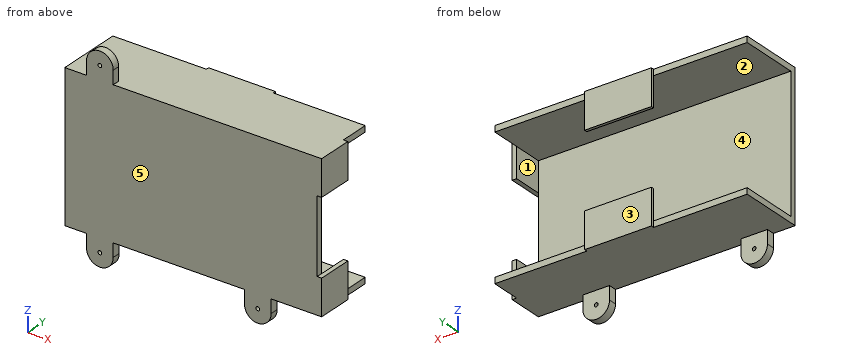
from build123d import *

# Parameters (mm, degrees)
SKETCH1_W           = 215.9
SKETCH1_H           = 114.3
BOSS_EXTRUDE1_DEPTH = 5.08
SKETCH2_W           = 215.9
SKETCH2_H           = 55.88
BOSS_EXTRUDE2_DEPTH = 5.08
SKETCH4_W           = 30.48
SKETCH4_H           = 30.48
BOSS_EXTRUDE3_DEPTH = 3.81
SKETCH5_W           = 57.15
SKETCH5_H           = 30.48
SKETCH5_W_2         = 57.169606557
BOSS_EXTRUDE4_DEPTH = 2.54
BOSS_EXTRUDE6_DEPTH = 15.875
SKETCH14_R          = 1.5875
CUT_EXTRUDE1_DEPTH  = 236.930487909
BOSS_EXTRUDE7_DEPTH = 15.875
SKETCH21_R          = 1.5875
CUT_EXTRUDE6_DEPTH  = 236.930487909
CUT_EXTRUDE10_START = -9.525
CUT_EXTRUDE10_DEPTH = 9.525
CUT_EXTRUDE11_START = -8.89
CUT_EXTRUDE11_DEPTH = 8.89
CUT_EXTRUDE12_START = -8.89
CUT_EXTRUDE12_DEPTH = 8.89


with BuildPart() as part:
    # Sketch1 → Boss-Extrude1 (new body)
    with BuildSketch(Plane(origin=(0, 0, 0), x_dir=(1, 0, 0), z_dir=(0, 1, 0))):
        with Locations((-107.95, 0)):
            Rectangle(SKETCH1_W, SKETCH1_H)
    extrude(amount=BOSS_EXTRUDE1_DEPTH)

    # Sketch2 → Boss-Extrude2 (add)
    with BuildSketch(Plane.XY.offset(57.15)):
        with Locations((-107.95, 27.94)):
            Rectangle(SKETCH2_W, SKETCH2_H)
    boss_extrude2 = extrude(amount=BOSS_EXTRUDE2_DEPTH)

    # Mirror1: Boss-Extrude2 across plane
    add(boss_extrude2.mirror(Plane.XY))

    # Sketch4 → Boss-Extrude3 (add)
    with BuildSketch(Plane(origin=(0, 0, 0), x_dir=(0, 0, -1), z_dir=(1, 0, 0))):
        with Locations((-46.99, 15.24)):
            Rectangle(SKETCH4_W, SKETCH4_H)
        with Locations((46.99, 15.24)):
            Rectangle(SKETCH4_W, SKETCH4_H)
    extrude(amount=BOSS_EXTRUDE3_DEPTH)

    # Sketch5 → Boss-Extrude4 (add)
    with BuildSketch(Plane(origin=(0, 55.88, 0), x_dir=(1, 0, 0), z_dir=(0, 1, 0))):
        with Locations((-107.309206557, 46.99)):
            Rectangle(SKETCH5_W, SKETCH5_H)
        with Locations((-107.299403278, -46.99)):
            Rectangle(SKETCH5_W_2, SKETCH5_H)
    extrude(amount=BOSS_EXTRUDE4_DEPTH)

    # Sketch12 → Boss-Extrude6 (add)
    with BuildSketch(Plane(origin=(0, 0, 0), x_dir=(1, 0, 0), z_dir=(0, 1, 0))):
        with BuildLine():
            Line((-62.23, 62.23), (-62.23, 73.66))
            ThreePointArc((-62.23, 73.66), (-50.8, 85.09), (-39.37, 73.66))
            Line((-39.37, 73.66), (-39.37, 62.23))
            Line((-39.37, 62.23), (-62.23, 62.23))
        make_face()
    extrude(amount=BOSS_EXTRUDE6_DEPTH)

    # Sketch14 → Cut-Extrude1 (cut, through all)
    with BuildSketch(Plane(origin=(0, 15.875, 0), x_dir=(1, 0, 0), z_dir=(0, 1, 0))):
        with Locations(Location((-50.8, 73.66, 0), (0, 0, 270))):
            Circle(SKETCH14_R)
    extrude(amount=-CUT_EXTRUDE1_DEPTH, mode=Mode.SUBTRACT)

    # Sketch20 → Boss-Extrude7 (add)
    with BuildSketch(Plane(origin=(0, 0, 0), x_dir=(1, 0, 0), z_dir=(0, 1, 0))):
        with BuildLine():
            Line((-197.317867116, 62.23), (-197.317867116, 73.66))
            ThreePointArc((-197.317867116, 73.66), (-185.887867116, 85.09), (-174.457867116, 73.66))
            Line((-174.457867116, 73.66), (-174.457867116, 62.23))
            Line((-174.457867116, 62.23), (-197.317867116, 62.23))
        make_face()
    boss_extrude7 = extrude(amount=BOSS_EXTRUDE7_DEPTH)

    # Sketch21 → Cut-Extrude6 (cut, through all)
    with BuildSketch(Plane(origin=(0, 15.875, 0), x_dir=(1, 0, 0), z_dir=(0, 1, 0))):
        with Locations(Location((-185.887867116, 73.66, 0), (0, 0, 270))):
            Circle(SKETCH21_R)
    cut_extrude6 = extrude(amount=-CUT_EXTRUDE6_DEPTH, mode=Mode.SUBTRACT)

    # Mirror4: Boss-Extrude7 across plane
    add(boss_extrude7.mirror(Plane.XY))

    # Mirror5: Cut-Extrude6 across plane
    add(cut_extrude6.mirror(Plane.XY), mode=Mode.SUBTRACT)

    # Sketch25 → Cut-Extrude10 (cut)
    with BuildSketch(Plane(origin=(0, 15.875, 0), x_dir=(1, 0, 0), z_dir=(0, 1, 0)).offset(CUT_EXTRUDE10_START)):
        with BuildLine():
            Line((-197.317867116, -62.23), (-197.317867116, -73.66))
            ThreePointArc((-197.317867116, -73.66), (-185.887867116, -85.09), (-174.457867116, -73.66))
            Line((-174.457867116, -73.66), (-174.457867116, -62.23))
            Line((-174.457867116, -62.23), (-197.317867116, -62.23))
        make_face()
    extrude(amount=CUT_EXTRUDE10_DEPTH, mode=Mode.SUBTRACT)

    # Sketch26 → Cut-Extrude11 (cut)
    with BuildSketch(Plane(origin=(0, 15.875, 0), x_dir=(1, 0, 0), z_dir=(0, 1, 0)).offset(CUT_EXTRUDE11_START)):
        with BuildLine():
            Line((-62.23, 62.23), (-39.37, 62.23))
            Line((-39.37, 62.23), (-39.37, 73.66))
            ThreePointArc((-39.37, 73.66), (-50.8, 85.09), (-62.23, 73.66))
            Line((-62.23, 73.66), (-62.23, 62.23))
        make_face()
    extrude(amount=CUT_EXTRUDE11_DEPTH, mode=Mode.SUBTRACT)

    # Sketch27 → Cut-Extrude12 (cut)
    with BuildSketch(Plane(origin=(0, 15.875, 0), x_dir=(1, 0, 0), z_dir=(0, 1, 0)).offset(CUT_EXTRUDE12_START)):
        with BuildLine():
            Line((-197.317867116, 62.23), (-174.457867116, 62.23))
            Line((-174.457867116, 62.23), (-174.457867116, 73.66))
            ThreePointArc((-174.457867116, 73.66), (-185.887867116, 85.09), (-197.317867116, 73.66))
            Line((-197.317867116, 73.66), (-197.317867116, 62.23))
        make_face()
    extrude(amount=CUT_EXTRUDE12_DEPTH, mode=Mode.SUBTRACT)


solid = part.part
Could you check a few things on this model? Use its own coordinates, in mm. Face numbers are marked on the shaded views. A direction names the side the tool comes from. Coordinates: 2 decimals unless noted, no trailing zeros. Order: outer loops, then holes, each group sorted by start corner. A loop starts at its lowest first (then second) coordinate and runs counter-clockwise, first axis right, second up. Notation, with made-up numbers: (-27, 74) -> (18, 74) arc R34 cw to (18, 108) -> close; hole circle Ø1 at (-18.5, -38.75). An arc over 180 degrees is marked (long way). One line per item, written item: value. Start each with the question number.
1) If I drill on L1, parallel to Z at x = -155, y = 46; L2, parallel to X at y = 4, z = -73.66; L3, parallel to X at y = 5.25, z = 73.66, over which ranges is the centre line in solid material (lowest first)? Write a range as [from, to].
2) I'm going to push flat-ended pins straight in: pin 1 (7.5 mm diameter, centred on y = 17.5, z = 48.5, fed in from -X); pin 2 (3 mm diameter, centred on y = 57.5, z = -42, fed in from -X); pin 3 (1.5 mm diameter, centred on x = -185, z = -59.5, fed in from +Y); pin 4 (3 mm diameter, centred on x = -185.89, z = -73.66, fed in from -Y). Where does each tip first touch, or does it pass through?
3) Imagine slicing it at A-A on z = 40.5. List the corners of the cut face in (x, y) for me.
4) Which directions (+Z, -Z, +X, -X, +Y, -Y) give clear straight access to the entire face, cutting with the end or side of a thin tool? Please do the marked faces 4 and 5.
5) Imagine slicing it at B-B on y = 35.5. List the corners of the cut face in (x, z) for me, plus the area to 3 significant figures.
6) We'd pull the mould along Z, two halves only. Please class the marked faces 1, 2 and 3: +Z half, -Z half, draft (parallel to the pull), parting line (faces both ways), or undercut.
7) Imagine slicing it at C-C on x = -93. List the corners of the cut face in (y, z) for me.
8) Imagine slicing it at D-D on z = -69. List the corners of the cut face in (x, y) for me (3 decimals), plus the area to 3 significant figures.
Answer list:
1. L1: z = [-62.23, -57.15], [57.15, 62.23]
1. L2: x = [-197.32, -187.48], [-184.3, -174.46], [-62.23, -52.39], [-49.21, -39.37]
1. L3: x = [-197.32, -187.48], [-184.3, -174.46]
2. pin 1: stops at x = 0
2. pin 2: stops at x = -135.88
2. pin 3: stops at y = 55.88
2. pin 4: passes through
3. outline: (-215.9, 0) -> (3.81, 0) -> (3.81, 30.48) -> (0, 30.48) -> (0, 5.08) -> (-215.9, 5.08) -> close; (-135.88, 55.88) -> (-78.71, 55.88) -> (-78.71, 58.42) -> (-135.88, 58.42) -> close
4. face 4: -X
4. face 5: +Z, -Z, +X, -X, -Y
5. outline: (-215.9, -62.23) -> (0, -62.23) -> (0, -57.15) -> (-215.9, -57.15) -> close; (-215.9, 57.15) -> (0, 57.15) -> (0, 62.23) -> (-215.9, 62.23) -> close
5. area: 2,190 mm2
6. face 1: undercut
6. face 2: undercut
6. face 3: draft
7. outline: (0, -62.23) -> (58.42, -62.23) -> (58.42, -31.75) -> (55.88, -31.75) -> (55.88, -57.15) -> (5.08, -57.15) -> (5.08, 57.15) -> (55.88, 57.15) -> (55.88, 31.75) -> (58.42, 31.75) -> (58.42, 62.23) -> (0, 62.23) -> close
8. outline: (-197.318, 0) -> (-174.458, 0) -> (-174.458, 6.985) -> (-197.318, 6.985) -> close; (-62.23, 0) -> (-39.37, 0) -> (-39.37, 6.985) -> (-62.23, 6.985) -> close
8. area: 319 mm2
